```python
from build123d import *

# Parameters (mm, degrees)
PAD039_DEPTH    = 10
SKETCH109_R     = 200
SKETCH109_R_2   = 164.5
POCKET046_DEPTH = 7
SKETCH110_R     = 200
SKETCH110_R_2   = 173.831445
POCKET047_DEPTH = 49.001
SKETCH107_R     = 2.75
POCKET048_DEPTH = 32


with BuildPart() as part:
    # Sketch108 → Pad039 (new body, symmetric)
    with BuildSketch(Plane.XY):
        with BuildLine():
            Line((-32, 15), (14.5, 15))
            ThreePointArc((17, 12.5), (16.267767, 14.267767), (14.5, 15))
            Line((17, 12.5), (17, -12.5))
            ThreePointArc((14.5, -15), (16.267767, -14.267767), (17, -12.5))
            Line((14.5, -15), (-32, -15))
            Line((-32, -15), (-32, 15))
        make_face()
        with BuildLine():
            Line((-11, 10.25), (11, 10.25))
            ThreePointArc((12, 9.25), (11.707107, 9.957107), (11, 10.25))
            Line((12, 9.25), (12, -9.25))
            ThreePointArc((11, -10.25), (11.707107, -9.957107), (12, -9.25))
            Line((11, -10.25), (-11, -10.25))
            ThreePointArc((-12, -9.25), (-11.707107, -9.957107), (-11, -10.25))
            Line((-12, -9.25), (-12, 9.25))
            ThreePointArc((-11, 10.25), (-11.707107, 9.957107), (-12, 9.25))
        make_face(mode=Mode.SUBTRACT)
    extrude(amount=PAD039_DEPTH, both=True)

    # Sketch109 (on DatumPlane) → Pocket046 (cut)
    with BuildSketch(Plane(origin=(-32, 0, 0), x_dir=(0, -1, 0), z_dir=(-1, 0, 0))):
        with Locations((0, 164.5)):
            Circle(SKETCH109_R)
        with Locations((0, 164.5)):
            Circle(SKETCH109_R_2, mode=Mode.SUBTRACT)
    extrude(amount=-POCKET046_DEPTH, mode=Mode.SUBTRACT)

    # Sketch110 (on DatumPlane) → Pocket047 (cut, through all)
    with BuildSketch(Plane(origin=(-32, 0, 0), x_dir=(0, -1, 0), z_dir=(-1, 0, 0))):
        with Locations((0, 165)):
            Circle(SKETCH110_R)
        with Locations((0, 165)):
            Circle(SKETCH110_R_2, mode=Mode.SUBTRACT)
    extrude(amount=-POCKET047_DEPTH, mode=Mode.SUBTRACT)

    # Sketch107 → Pocket048 (cut)
    with BuildSketch(Plane.YZ.offset(18)):
        Circle(SKETCH107_R)
    extrude(amount=-POCKET048_DEPTH, mode=Mode.SUBTRACT)


with BuildPart() as part_1:
    # Body022022 placement: moved
    add(part.part.moved(Location((157, 0, -82))))


solid = part_1.part
```
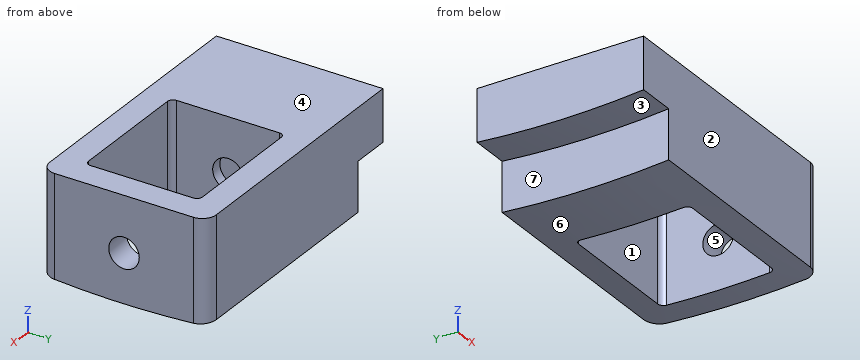
For this review, take the finished solid that the model builds, in its own axes (mm). Face numbers are marked on the shaded views. A direction names the side the tool comes from. Round coordinates to 2 decimals unless told otherwise and drop trailing zeros. Write each loop counter-clockwise with the first axis right and the second up, starting at its lowest first coordinate (ties: lowest second). Pieces come first, ordered by that corner, then holes. Notation, with made-up numbers: (76, 78.25) -> (132, 78.25) arc R15 ccw to (132, 92.25) -> close; hole circle Ø7 at (-21, -35). An arc over 180 degrees is marked (long way). Use one line per item in the form item = value.
Q1. Consider section B-B (y = 0). State the section outline as (x, z) points, then the cut area to 3 significant figures.
Resolved:
outline = (125, -82) -> (132, -82) -> (132, -90.83) -> (145, -90.83) -> (145, -84.75) -> (143, -84.75) -> (143, -79.25) -> (145, -79.25) -> (145, -72) -> (125, -72) -> close; (169, -90.83) -> (174, -90.83) -> (174, -84.75) -> (169, -84.75) -> close; (169, -79.25) -> (174, -79.25) -> (174, -72) -> (169, -72) -> close
area = 370 mm²
Q2. Machinability: for the marked faces 1, 2 and 3, which of the approach directions +Z, -Z, +X, -X, +Y, -Y give a long, thin tool a straight path to every point of the face, cutting with its end or side? Answer none if there is none.
Resolved:
face_1 = +Z, -Z
face_2 = +Z, -Z, +X, -X, -Y
face_3 = -Z, -X
Q3. Consider section C-C (z = -85.5). State the section outline as (x, y) points, then the cut area to 3 significant figures.
Resolved:
outline = (132, -15) -> (171.5, -15) arc R2.5 ccw to (174, -12.5) -> (174, 12.5) arc R2.5 ccw to (171.5, 15) -> (132, 15) -> close; hole (145, -9.25) arc R1 ccw to (146, -10.25) -> (168, -10.25) arc R1 ccw to (169, -9.25) -> (169, 9.25) arc R1 ccw to (168, 10.25) -> (146, 10.25) arc R1 ccw to (145, 9.25) -> close
area = 766 mm²
Q4. Clearance check with flat-ended pins moving along their axes: pin 1 Ø3 at (y, z) = (-0.5, -86) entering from -X; pin 2 Ø6.5 at (y, z) = (0, -82) entering from +X; pin 3 Ø1.6 at (y, z) = (-0.5, -83) entering from +X. State where each tip first meets the part, or that it passes through.
Resolved:
pin_1 = 132
pin_2 = 174
pin_3 = 143
Q5. The part is to be moulded in two halves that separate along Z. For the marked faces 4, 5, 6 and 7, say which applies: released by +Z, released by -Z, zero draft, split by the parting line, or undercut.
Resolved:
face_4 = released by +Z
face_5 = undercut
face_6 = released by -Z
face_7 = zero draft
Q6. Consider section D-D (y = 3.5). State the section outline as (x, z) points, then the cut area to 3 significant figures.
Resolved:
outline = (125, -81.96) -> (132, -81.96) -> (132, -90.8) -> (145, -90.8) -> (145, -72) -> (125, -72) -> close; (169, -90.8) -> (174, -90.8) -> (174, -72) -> (169, -72) -> close
area = 408 mm²
Q7. To check wall thickness, follow probe 1 along Z at (x, y) = (173, 0); probe 2 along Y at (x, z) = (155.5, -76.25); probe 3 along X at (y, z) = (0.5, -88.5). State the ranges of each line that lie inside material, in increasing order. Write a range as from..to.
Resolved:
probe_1 = -90.83..-84.75, -79.25..-72
probe_2 = -15..-10.25, 10.25..15
probe_3 = 132..145, 169..174
Q8. Consider section A-A (x = 163.5). State the section outline as (y, z) points, then the cut area to 3 significant figures.
Resolved:
outline = (-15, -90.18) arc R173.83 ccw to (-10.25, -90.53) -> (-10.25, -72) -> (-15, -72) -> close; (10.25, -90.53) arc R173.83 ccw to (15, -90.18) -> (15, -72) -> (10.25, -72) -> close
area = 174 mm²
